Verification items for this drawing (mm, ordinates from the low corner). A direction names the side the tool comes from. Coordinates: 2 decimals unless noted, no trailing zeros. Loops run counter-clockwise (first coordinate to the right, second up) from the corner with the lowest first, then second, coordinate; pieces in that order, holes last. Notation, with made-up numbers: M -20.75,-16.5 L 8.25,-16.5 A10 ccw 8.25,2.5 Z; hole C -33,85 d4. An arc over 180 degrees is marked long. Return JSON: item names as keys, results as strings.
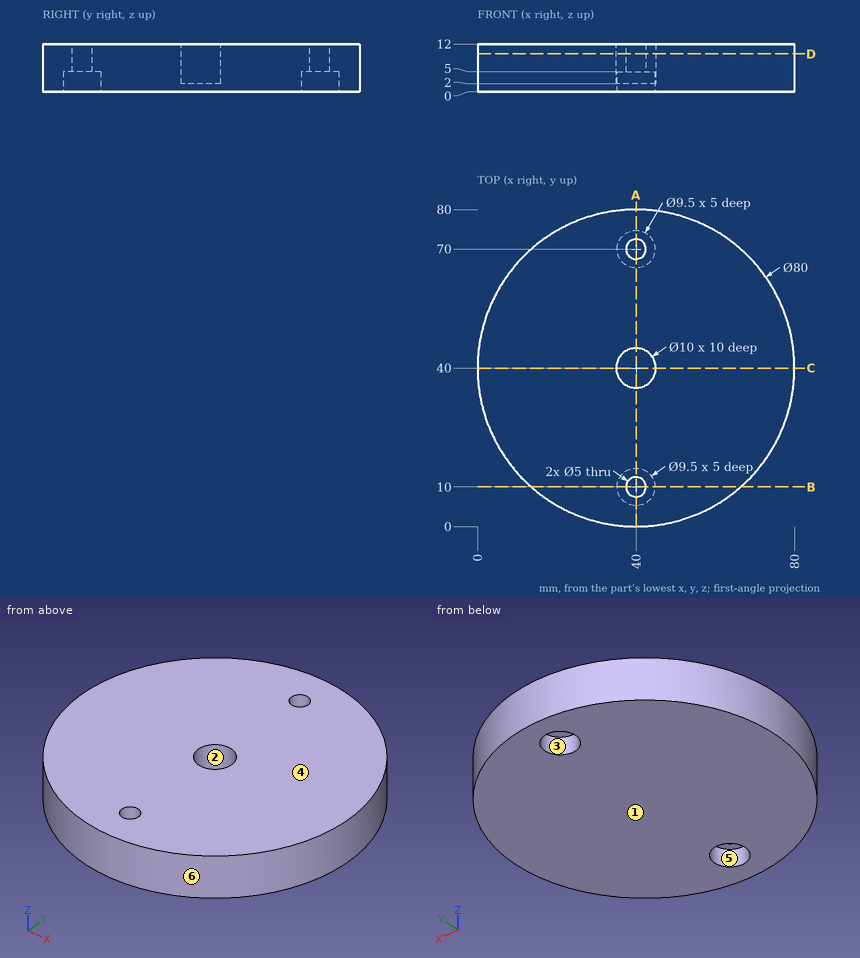
1) Section check B-B on y = 10. Record the cut outline in (x, z), then the cut area to 3 significant figures.
Answers:
{"outline": "M 13.54,0 L 35.25,0 L 35.25,5 L 37.5,5 L 37.5,12 L 13.54,12 Z; M 42.5,5 L 44.75,5 L 44.75,0 L 66.46,0 L 66.46,12 L 42.5,12 Z", "area": "552 mm²"}
2) Scan lines: line 1 along Y through (x, z) = (40, 5.5); line 2 along Y through (x, z) = (40, 3.2); line 3 along X through (y, z) = (12.5, 2.75). Record each from-to range of solid material in increasing order. Write a range as [from, to].
Answers:
{"line 1": "[0, 7.5], [12.5, 35], [45, 67.5], [72.5, 80]", "line 2": "[0, 5.25], [14.75, 35], [45, 65.25], [74.75, 80]", "line 3": "[10.95, 35.96], [44.04, 69.05]"}
3) Draft check along Y on the marked faces 4, 5 and 6. Enter one of: +Y half, -Y half, draft (parallel to the pull), parting line (faces both ways), or undercut.
Answers:
{"face 4": "draft", "face 5": "undercut", "face 6": "parting line"}
4) Section check D-D on z = 9.5. Record the cut outline in (x, y), then the cut area to 3 significant figures.
Answers:
{"outline": "C 40,40 d80; hole C 40,40 d10; hole C 40,10 d5; hole C 40,70 d5", "area": "4,910 mm²"}
5) Set-up check for the marked faces 1, 2 and 3: record each of +Z, -Z, +X, -X, +Y, -Y from which the full face is reachable in a straight line by a thin tool's end or side.
Answers:
{"face 1": "-Z, +X, -X, +Y, -Y", "face 2": "+Z", "face 3": "-Z"}
6) Section check A-A on x = 40. Record the cut outline in (y, z).
Answers:
{"outline": "M 0,0 L 5.25,0 L 5.25,5 L 7.5,5 L 7.5,12 L 0,12 Z; M 12.5,5 L 14.75,5 L 14.75,0 L 65.25,0 L 65.25,5 L 67.5,5 L 67.5,12 L 45,12 L 45,2 L 35,2 L 35,12 L 12.5,12 Z; M 72.5,5 L 74.75,5 L 74.75,0 L 80,0 L 80,12 L 72.5,12 Z"}
7) Section check C-C on y = 40. Record the cut outline in (x, z), then the cut area to 3 significant figures.
Answers:
{"outline": "M 0,0 L 80,0 L 80,12 L 45,12 L 45,2 L 35,2 L 35,12 L 0,12 Z", "area": "860 mm²"}
8) Go/stop test with flat-tipped pins: pin 1 Ø2 at (x, z) = (61, 4) entering from -Y; pin 2 Ø6.5 at (x, y) = (40, 10) entering from -Z; pin 3 Ø4 at (y, z) = (12.5, 9.5) entering from +X. Record where each tip stops, or that it passes through.
Answers:
{"pin 1": "y = 5.36", "pin 2": "z = 5", "pin 3": "x = 70.82"}
